from build123d import *

# Parameters (mm, degrees)
SKETCH1_W           = 25
SKETCH1_H           = 211.5
BOSS_EXTRUDE1_DEPTH = 10
SKETCH2_W           = 10
SKETCH2_H           = 15
SKETCH2_H_2         = 10
SKETCH2_W_2         = 191.5
BOSS_EXTRUDE2_DEPTH = 45
SKETCH3_3_W         = 185
SKETCH3_3_H         = 3.5
BOSS_EXTRUDE4_DEPTH = 10
CUT_EXTRUDE11_REACH = 222.795
SKETCH15_R          = 1.9
LPATTERN2_COUNT     = 3
LPATTERN2_PITCH     = 88.5
SKETCH16_W          = 185
SKETCH16_H          = 3.5
SKETCH16_W_2        = 184.8
SKETCH16_H_2        = 3.3
CUT_EXTRUDE12_DEPTH = 10
CUT_EXTRUDE13_REACH = 222.821
SKETCH17_W          = 184.8
SKETCH17_H          = 0.2
CUT_EXTRUDE3_REACH  = 225.983
BOSS_EXTRUDE3_REACH = 224.671
CUT_EXTRUDE4_REACH  = 224.671
SKETCH10_W          = 78.5
SKETCH10_H          = 0.625
SKETCH10_W_2        = 113
SKETCH4_W           = 3.5
SKETCH4_H           = 34
CUT_EXTRUDE2_DEPTH  = 5
CUT_EXTRUDE5_DEPTH  = 5
SKETCH12_W          = 78.5
SKETCH12_H          = 5
CUT_EXTRUDE6_DEPTH  = 14.375
CUT_EXTRUDE7_REACH  = 224.671
SKETCH9_R           = 1.9
CUT_EXTRUDE9_DEPTH  = 2.5
LPATTERN1_COUNT     = 2
LPATTERN1_PITCH     = 64


with BuildPart() as part:
    # Sketch1 → Boss-Extrude1 (new body)
    with BuildSketch(Plane(origin=(0, 0, 0), x_dir=(0, 1, 0), z_dir=(0, 0, 1))):
        with Locations((12.5, 105.75)):
            Rectangle(SKETCH1_W, SKETCH1_H)
    boss_extrude1 = extrude(amount=BOSS_EXTRUDE1_DEPTH)

    # Sketch2 → Boss-Extrude2 (add)
    with BuildSketch(Plane.XY.offset(10)):
        with Locations((-5, 7.5)):
            Rectangle(SKETCH2_W, SKETCH2_H)
        with Locations((-5, 20)):
            Rectangle(SKETCH2_W, SKETCH2_H_2)
        with Locations((-105.75, 20)):
            Rectangle(SKETCH2_W_2, SKETCH2_H_2)
        with Locations((-206.5, 20)):
            Rectangle(SKETCH2_W, SKETCH2_H_2)
        with Locations((-206.5, 7.5)):
            Rectangle(SKETCH2_W, SKETCH2_H)
    extrude(amount=BOSS_EXTRUDE2_DEPTH)

    # Mirror1: Boss-Extrude1 across plane
    add(boss_extrude1.mirror(Plane.XY.offset(32.5)))

    # Sketch3<3> → Boss-Extrude4 (add)
    with BuildSketch(Plane.XZ):
        with Locations((-105.75, 5)):
            Rectangle(SKETCH3_3_W, SKETCH3_3_H)
    extrude(amount=BOSS_EXTRUDE4_DEPTH)

    # Sketch15 → Cut-Extrude11 (cut, up to next)
    with BuildSketch(Plane(origin=(0, 0, 6.75), x_dir=(-1, 0, 0), z_dir=(0, 0, 1)), mode=Mode.PRIVATE) as cut_extrude11_sk1:
        with Locations(Location((194.25, 5, 0), (0, 0, 180))):
            Circle(SKETCH15_R)
    cut_extrude11_tool1 = extrude(cut_extrude11_sk1.sketch, amount=-CUT_EXTRUDE11_REACH, mode=Mode.PRIVATE) & part.part
    cut_extrude11 = cut_extrude11_tool1.solids().sort_by_distance((-194.25, -5, 6.75))[0]
    add(cut_extrude11, mode=Mode.SUBTRACT)

    # LPattern2: Cut-Extrude11 ×3
    with Locations(*[(i * LPATTERN2_PITCH, 0, 0) for i in range(1, LPATTERN2_COUNT)]):
        add(cut_extrude11, mode=Mode.SUBTRACT)

    # Sketch16 → Cut-Extrude12 (cut)
    with BuildSketch(Plane.XZ.offset(10)):
        with Locations((-105.75, 5)):
            Rectangle(SKETCH16_W, SKETCH16_H)
        with Locations((-105.75, 5)):
            Rectangle(SKETCH16_W_2, SKETCH16_H_2, mode=Mode.SUBTRACT)
    extrude(amount=-CUT_EXTRUDE12_DEPTH, mode=Mode.SUBTRACT)

    # Sketch17 → Cut-Extrude13 (cut, up to next)
    with BuildSketch(Plane(origin=(0, 0, 6.65), x_dir=(-1, 0, 0), z_dir=(0, 0, 1)), mode=Mode.PRIVATE) as cut_extrude13_sk1:
        with Locations((105.75, 9.9)):
            Rectangle(SKETCH17_W, SKETCH17_H)
    cut_extrude13_tool1 = extrude(cut_extrude13_sk1.sketch, amount=-CUT_EXTRUDE13_REACH, mode=Mode.PRIVATE) & part.part
    add(cut_extrude13_tool1.solids().sort_by_distance((-105.75, -9.9, 6.65))[0], mode=Mode.SUBTRACT)

    # Sketch5 → Cut-Extrude3 (cut, up to next)
    with BuildSketch(Plane(origin=(0, 25, 0), x_dir=(-1, 0, 0), z_dir=(0, 1, 0)), mode=Mode.PRIVATE) as cut_extrude3_sk1:
        Polygon((0, 65), (0, 39), (10, 39), (123, 65), align=None)
    cut_extrude3_tool1 = extrude(cut_extrude3_sk1.sketch, amount=-CUT_EXTRUDE3_REACH, mode=Mode.PRIVATE) & part.part
    add(cut_extrude3_tool1.solids().sort_by_distance((-41.250627, 25, 55.681704))[0], mode=Mode.SUBTRACT)

    # Sketch7 → Boss-Extrude3 (add, up to next)
    with BuildSketch(Plane.XZ, mode=Mode.PRIVATE) as boss_extrude3_sk1:
        Polygon((-10, 39), (-123, 65), (-123, 55), (-10, 29), align=None)
    boss_extrude3_tool1 = extrude(boss_extrude3_sk1.sketch, amount=-BOSS_EXTRUDE3_REACH, mode=Mode.PRIVATE) - part.part
    add(boss_extrude3_tool1.solids().sort_by_distance((-66.5, 0, 47))[0])

    # Sketch10 → Cut-Extrude4 (cut, up to next)
    with BuildSketch(Plane.XY.offset(65), mode=Mode.PRIVATE) as cut_extrude4_sk1:
        with Locations((-162.25, 0.3125)):
            Rectangle(SKETCH10_W, SKETCH10_H)
    cut_extrude4_tool1 = extrude(cut_extrude4_sk1.sketch, amount=-CUT_EXTRUDE4_REACH, mode=Mode.PRIVATE) & part.part
    # Sketch10 → Cut-Extrude4 (cut, up to next)
    with BuildSketch(Plane.XY.offset(65), mode=Mode.PRIVATE) as cut_extrude4_sk2:
        with Locations((-66.5, 0.3125)):
            Rectangle(SKETCH10_W_2, SKETCH10_H)
    cut_extrude4_tool2 = extrude(cut_extrude4_sk2.sketch, amount=-CUT_EXTRUDE4_REACH, mode=Mode.PRIVATE) & part.part
    add(cut_extrude4_tool1.solids().sort_by_distance((-162.25, 0.3125, 65))[0], mode=Mode.SUBTRACT)
    add(cut_extrude4_tool2.solids().sort_by_distance((-66.5, 0.3125, 65))[0], mode=Mode.SUBTRACT)

    # Sketch4 → Cut-Extrude2 (cut)
    with BuildSketch(Plane.XZ):
        with Locations((-5, 22)):
            Rectangle(SKETCH4_W, SKETCH4_H)
    extrude(amount=-CUT_EXTRUDE2_DEPTH, mode=Mode.SUBTRACT)

    # Sketch11 → Cut-Extrude5 (cut)
    with BuildSketch(Plane.XZ):
        Polygon((-208.25, 15), (-208.25, 5), (-204.75, 5), (-204.75, 15), (-204.75, 65), (-208.25, 65), align=None)
    extrude(amount=-CUT_EXTRUDE5_DEPTH, mode=Mode.SUBTRACT)

    # Sketch12 → Cut-Extrude6 (cut)
    with BuildSketch(Plane.XZ.offset(-0.625)):
        with Locations((-162.25, 57.5)):
            Rectangle(SKETCH12_W, SKETCH12_H)
    extrude(amount=-CUT_EXTRUDE6_DEPTH, mode=Mode.SUBTRACT)

    # Sketch9 → Cut-Extrude7 (cut, up to next)
    with BuildSketch(Plane.XY.offset(65), mode=Mode.PRIVATE) as cut_extrude7_sk1:
        with Locations((-194.25, 5.625)):
            Circle(SKETCH9_R)
    cut_extrude7_tool1 = extrude(cut_extrude7_sk1.sketch, amount=-CUT_EXTRUDE7_REACH, mode=Mode.PRIVATE) & part.part
    cut_extrude7 = cut_extrude7_tool1.solids().sort_by_distance((-194.25, 5.625, 65))[0]
    add(cut_extrude7, mode=Mode.SUBTRACT)

    # Sketch13 → Cut-Extrude9 (cut)
    with BuildSketch(Plane(origin=(0, 0, 60), x_dir=(1, 0, 0), z_dir=(0, 0, -1))):
        Polygon((-192.297927406, -9.006088913), (-190.345854812, -5.625), (-192.297927406, -2.243911087), (-196.202072594, -2.243911087), (-198.154145188, -5.625), (-196.202072594, -9.006088913), align=None)
    cut_extrude9 = extrude(amount=-CUT_EXTRUDE9_DEPTH, mode=Mode.SUBTRACT)

    # LPattern1: Cut-Extrude7, Cut-Extrude9 ×2
    with Locations(*[(i * LPATTERN1_PITCH, 0, 0) for i in range(1, LPATTERN1_COUNT)]):
        add(cut_extrude7, mode=Mode.SUBTRACT)
        add(cut_extrude9, mode=Mode.SUBTRACT)


solid = part.part
Design review of the part built by this model. Coordinates are the model's own, in mm. A direction names the side the tool comes from. Give positions to 0.01 mm unless a question says otherwise; leave off trailing zeros. Loops run counter-clockwise (first coordinate to the right, second up) from the corner with the lowest first, then second, coordinate; pieces in that order, holes last. Notation, with made-up numbers: (40.5, -0.5) -> (53.5, -0.5) arc R12 ccw to (53.5, 17.5) -> close; hole circle Ø2 at (49, -5). An arc over 180 degrees is marked (long way). One line per question, with ' | ' between items. Start each with the question number.
(1) For line 1 (X direction, y = 3.5, z = 8); line 2 (X direction, y = 3.5, z = 18.5); line 3 (Y direction, x = -194.25, z = 5.75), list the stretches that pass through material, from the lowest coordinate up.
(2) We need section D-D (x = -194.25). State the section outline as (y, z) points (3 decimals).
(3) We need section C-C (z = 12). State the section outline as (x, y) points, and give its area (3 significant figures).
(4) We need section A-A (y = 11.5). State the section outline as (x, z) points, and give its area (3 significant figures).
(5) We need section B-B (x = -17.25). State the section outline as (y, z) points (3 decimals), and give its area (3 significant figures).
(6) For faces 5 (the face through (-193, 4, 62.5)), 6 (the face through (-208.25, 2, 35)), 7 (the face through (-201.5, 7, 38)), list the 3-axis set-ups (+Z, -Z, +X, -X, +Y, -Y) from which the entire face can be reached by the end or side of a thin tool; tool diameter is ignored.
(7) Insertion check: P1, Ø6, axis at x = -138, y = -5, coming from the +Z side; P2, Ø18, axis at x = -120.5, z = 55.5, coming from the -Y side (3 decimals); P3, Ø1.8, axis at x = -207, y = 3, coming from the +Z side. Each pin has a flat end and moves straight along its axis. Give the tip position at first contact, or say it passes through.
(8) Draft analysis for pull direction Z (two halves, no side actions). For faces 1 (the face through (-10, 7, 21)), 2 (the face through (-196.15, -4.92, 5.02)), 3 (the face through (-65.71, 12.64, 51.82)), 4 (the face through (-107, 12, 0)), state which applies: +Z half, -Z half, draft (parallel to the pull), parting line (faces both ways), or undercut.
The answers:
1) line 1: x = -211.5 to -208.25, -204.75 to -6.75, -3.25 to 0 | line 2: x = -211.5 to -208.25, -204.75 to -201.5, -10 to -6.75, -3.25 to 0 | line 3: y = -9.8 to -6.9, -3.1 to 25
2) outline: (-9.8, 3.35) -> (-6.9, 3.35) -> (-6.9, 6.65) -> (-9.8, 6.65) -> close; (-3.1, 3.35) -> (0, 3.35) -> (0, 0) -> (25, 0) -> (25, 65) -> (7.525, 65) -> (7.525, 62.5) -> (9.006, 62.5) -> (9.006, 60) -> (15, 60) -> (15, 10) -> (0, 10) -> (0, 6.65) -> (-3.1, 6.65) -> close; (0.625, 60) -> (2.244, 60) -> (2.244, 62.5) -> (3.725, 62.5) -> (3.725, 65) -> (0.625, 65) -> close
3) outline: (-211.5, 0) -> (-208.25, 0) -> (-208.25, 5) -> (-204.75, 5) -> (-204.75, 0) -> (-201.5, 0) -> (-201.5, 15) -> (-10, 15) -> (-10, 0) -> (-6.75, 0) -> (-6.75, 5) -> (-3.25, 5) -> (-3.25, 0) -> (0, 0) -> (0, 25) -> (-211.5, 25) -> close | area: 2,380 mm^2
4) outline: (-211.5, 0) -> (0, 0) -> (0, 39) -> (-10, 39) -> (-123, 65) -> (-211.5, 65) -> close; hole (-201.5, 10) -> (-10, 10) -> (-10, 29) -> (-123, 55) -> (-123, 60) -> (-201.5, 60) -> close | area: 4,480 mm^2
5) outline: (-9.8, 3.35) -> (-6.9, 3.35) -> (-6.9, 6.65) -> (-9.8, 6.65) -> close; (-3.1, 3.35) -> (0, 3.35) -> (0, 0) -> (25, 0) -> (25, 40.668) -> (0.625, 40.668) -> (0.625, 30.668) -> (15, 30.668) -> (15, 10) -> (0, 10) -> (0, 6.65) -> (-3.1, 6.65) -> close | area: 720 mm^2
6) face 5: none | face 6: +Z, -Y | face 7: -Y
7) P1: stops at z = 6.65 | P2: stops at y = 0.625 | P3: stops at z = 5
8) face 1: undercut | face 2: draft | face 3: +Z half | face 4: -Z half
